Input: part model. Units: mm. Frame: model coordinates. Coordinates: 2 decimals unless noted, no trailing zeros. Loops run counter-clockwise (first coordinate to the right, second up) from the corner with the lowest first, then second, coordinate; pieces in that order, holes last.
Item 1: Ray query, line 1 along Y through (x, z) = (4, 2203.5); line 2 along Z through (x, y) = (38.5, -30). Return the intervals inside material, ascending.
Item 2: Pull-direction query (Y, two-part tool) for faces 1 (the flat face through (0, 0, 534)), 2 (the flat face through (-1, 22.5, 1943)), 3 (the flat face through (5.82, -35.792, 3327.416)), 4 (the flat face through (5.8, -35.4, 3322.4)); classes: released by +Y, released by -Y, zero draft, split by the parting line, or undercut.
Item 3: Contact query for flat-ended pins moving along their axis: P1, Ø5, axis at x = -59, y = 5, coming from the +Z side; P2, Ø10, axis at x = 39.5, y = -27.5, coming from the -Z side; P3, Ø4, axis at y = -11.5, z = 2205.5, coming from the -X side. Output: stop coordinate, or through.
Item 4: Section A-A on z = 1401.5. Return loops of the section in (x, y).
```python
from build123d import *

# Parameters (mm, degrees)
F0_W      = 45
F0_H      = 45
F1_DEPTH  = 3330
F6_W      = 45
F6_H      = 45.842251273
F7_DEPTH  = 25
F8_W      = 60
F8_H      = 60
F8_W_2    = 90
F8_H_2    = 90
F9_DEPTH  = 5
F10_R     = 6
F11_DEPTH = 25
F12_W     = 150
F12_H     = 4.7702248844
F13_DEPTH = 3358.6871623993
F15_DEPTH = 111
F16_W     = 45
F16_H     = 45
F17_DEPTH = 534


with BuildPart() as f1:
    # F0 (on Top) → F1 (new body)
    with BuildSketch(Plane.XY):
        Rectangle(F0_W, F0_H)
    extrude(amount=F1_DEPTH)

    # F6 (on face) → F7 (join)
    with BuildSketch(Plane(origin=(0, -624.5391596736, 3212.9754420296), x_dir=(1, 0, 0), z_dir=(0, 0.1908089954, -0.9816271834))):
        with Locations((0, -636.2284686128)):
            Rectangle(F6_W, F6_H)
    extrude(amount=F7_DEPTH)

    # F8 (on face) → F9 (join)
    with BuildSketch(Plane(origin=(0, -624.5391596736, 3212.9754420296), x_dir=(1, 0, 0), z_dir=(0, 0.1908089954, -0.9816271834))):
        with Locations((7.5, -629.1495942493)):
            Rectangle(F8_W, F8_H)
        with Locations((-67.5, -629.1495942493)):
            Rectangle(F8_W_2, F8_H)
        with Locations((82.5, -629.1495942493)):
            Rectangle(F8_W_2, F8_H)
        with Locations((7.5, -554.1495942493)):
            Rectangle(F8_W, F8_H_2)
    extrude(amount=F9_DEPTH)

    # F10 (on face) → F11 (cut)
    with BuildSketch(Plane(origin=(0, -624.5391596736, 3212.9754420296), x_dir=(1, 0, 0), z_dir=(0, -0.1908089954, 0.9816271834))):
        with BuildLine():
            ThreePointArc((22.5, 540.1495942493), (18.2573593129, 529.9069535622), (28.5, 534.1495942493))
            Line((28.5, 534.1495942493), (22.5, 534.1495942493))
            Line((22.5, 534.1495942493), (22.5, 540.1495942493))
        make_face()
        with BuildLine():
            Line((22.5, 534.1495942493), (28.5, 534.1495942493))
            ThreePointArc((28.5, 534.1495942493), (26.7426406871, 538.3922349364), (22.5, 540.1495942493))
            Line((22.5, 540.1495942493), (22.5, 534.1495942493))
        make_face()
        with BuildLine():
            ThreePointArc((28.5, 574.1495942493), (18.2573593129, 578.3922349364), (22.5, 568.1495942493))
            ThreePointArc((22.5, 568.1495942493), (26.7426406871, 569.9069535622), (28.5, 574.1495942493))
        make_face()
        with BuildLine():
            ThreePointArc((96.5, 614.1495942493), (98.2573593129, 609.9069535622), (102.5, 608.1495942493))
            Line((102.5, 608.1495942493), (102.5, 614.1495942493))
            Line((102.5, 614.1495942493), (96.5, 614.1495942493))
        make_face()
        with Locations((62.5, 614.1495942493)):
            Circle(F10_R)
        with BuildLine():
            Line((102.5, 614.1495942493), (102.5, 608.1495942493))
            ThreePointArc((102.5, 608.1495942493), (106.7426406871, 609.9069535622), (108.5, 614.1495942493))
            ThreePointArc((108.5, 614.1495942493), (102.5, 620.1495942493), (96.5, 614.1495942493))
            Line((96.5, 614.1495942493), (102.5, 614.1495942493))
        make_face()
        with Locations((-47.5, 614.1495942493)):
            Circle(F10_R)
        with Locations((-87.5, 614.1495942493)):
            Circle(F10_R)
    extrude(amount=-F11_DEPTH, mode=Mode.SUBTRACT)

    # F12 (on Top) → F13 (cut)
    with BuildSketch(Plane.XY):
        with Locations((52.5, 24.8851124422)):
            Rectangle(F12_W, F12_H)
    extrude(amount=F13_DEPTH, mode=Mode.SUBTRACT)

    # F14 (on face) → F15 (cut)
    with BuildSketch(Plane.YZ.offset(-22.5)):
        Polygon((22.5, 3333.6535304364), (23.4540449769, 3333.838977994), (22.5, 3338.7471139112), align=None)
    extrude(amount=-F15_DEPTH, mode=Mode.SUBTRACT)

    # F16 (on face) → F17 (cut)
    with BuildSketch(Plane(origin=(0, 0, 0), x_dir=(1, 0, 0), z_dir=(0, 0, -1))):
        Rectangle(F16_W, F16_H)
    extrude(amount=-F17_DEPTH, mode=Mode.SUBTRACT)


solid = f1.part
```
Results found:
1. line 1: y = -22.5 to 22.5
1. line 2: z = 3323.45 to 3328.54
2. face 1: zero draft
2. face 2: released by +Y
2. face 3: released by -Y
2. face 4: undercut
3. P1: stops at z = 3335.83
3. P2: stops at z = 3322.96
3. P3: stops at x = -22.5
4. outline: (-22.5, -22.5) - (22.5, -22.5) - (22.5, 22.5) - (-22.5, 22.5) - close
